Print and shaded views of the part. All mm, measured from the part's lowest x, y and z. A direction names the side the tool comes from. Round coordinates to 2 decimals unless told otherwise and drop trailing zeros. Loops run counter-clockwise (first coordinate to the right, second up) from the corner with the lowest first, then second, coordinate; pieces in that order, holes last. Notation, with made-up numbers: (51, -39) -> (62, -39) arc R17 cw to (62, -26) -> close; hole circle Ø7 at (-17, 35.25). An arc over 180 degrees is marked (long way). Use a Markdown table: item, result.
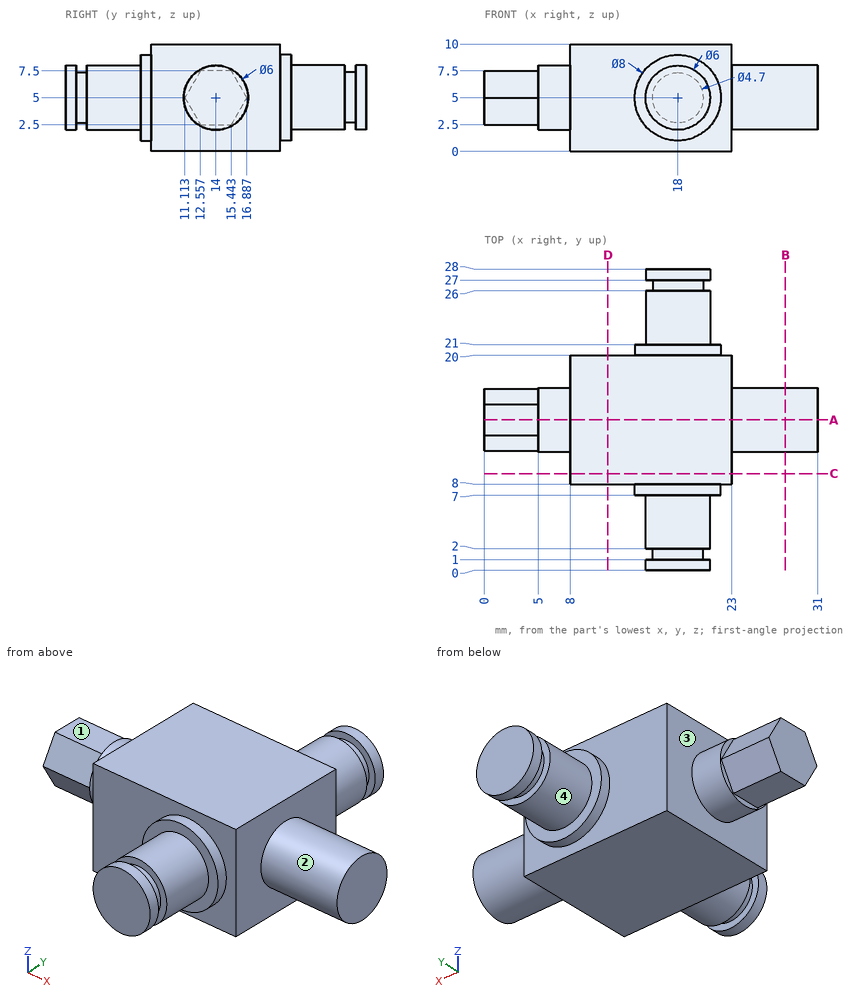
Q1. Flat gauge pins, fed straight in: pin 1 (1.4 mm diameter, centred on x = 3.5, y = 14.5, fed in from -Z); pin 2 (2 mm diameter, centred on x = 26.5, z = 2, fed in from -Y) (1 decimal); pin 3 (1.5 mm diameter, centred on y = 22, z = 1, fed in from -X); pin 4 (1.4 mm diameter, centred on x = 1.5, y = 14.5, fed in from +Z). Where does each tip first touch, or does it go through?
Results list:
| item | result |
|---|---|
| pin 1 | stops at z = 2.5 |
| pin 2 | stops at y = 11.8 |
| pin 3 | passes through |
| pin 4 | stops at z = 7.5 |
Q2. Drill centre lines: L1, parallel to Y at x = 9.5, z = 5.25; L2, parallel to X at y = 17, z = 6; L3, parallel to Y at x = 18.5, z = 8. Where is each one in solid material? Low to high. Write a range as from..to.
Results list:
| item | result |
|---|---|
| L1 | y = 8..20 |
| L2 | x = 8..23 |
| L3 | y = 7..21 |
Q3. Band-saw the part on C-C, the plane y = 9. Give the cut face in (x, z).
Results list:
| item | result |
|---|---|
| outline | (8, 0) -> (23, 0) -> (23, 10) -> (8, 10) -> close |
Q4. Band-saw the part on B-B, the plane x = 28. Give the cut face in (y, z).
Results list:
| item | result |
|---|---|
| outline | circle Ø6 at (14, 5) |
Q5. Tool access for the marked faces 1, 2, 3 and 4: list every direction of +Z, -Z, +X, -X, +Y, -Y with a clear straight run to the whole face (end or side of a thin tool).
Results list:
| item | result |
|---|---|
| face 1 | +Z, -X, +Y, -Y |
| face 2 | +X |
| face 3 | -X |
| face 4 | +Y |
Q6. Band-saw the part on A-A, the plane y = 14. Give the cut face in (x, z).
Results list:
| item | result |
|---|---|
| outline | (0, 2.5) -> (5, 2.5) -> (5, 2) -> (8, 2) -> (8, 0) -> (23, 0) -> (23, 2) -> (31, 2) -> (31, 8) -> (23, 8) -> (23, 10) -> (8, 10) -> (8, 8) -> (5, 8) -> (5, 7.5) -> (0, 7.5) -> close |
Q7. Band-saw the part on D-D, the plane x = 11.5. Give the cut face in (y, z).
Results list:
| item | result |
|---|---|
| outline | (8, 0) -> (20, 0) -> (20, 10) -> (8, 10) -> close |
